```python
from build123d import *

# Parameters (mm, degrees)
SKETCH1_W           = 34
SKETCH1_H           = 30
BOSS_EXTRUDE1_DEPTH = 22.2
CUT_EXTRUDE1_DEPTH  = 51.486037674
SKETCH3_R           = 4
CUT_EXTRUDE2_DEPTH  = 51.486037674


with BuildPart() as part:
    # Sketch1 → Boss-Extrude1 (new body)
    with BuildSketch(Plane(origin=(0, 0, 0), x_dir=(1, 0, 0), z_dir=(0, 1, 0))):
        with Locations((17, 15)):
            Rectangle(SKETCH1_W, SKETCH1_H)
    extrude(amount=BOSS_EXTRUDE1_DEPTH)

    # Sketch2 → Cut-Extrude1 (cut, through all)
    with BuildSketch(Plane.XY):
        Polygon((34, 17.6), (27, 17.6), (23.985037314, 22.2), (34, 22.2), align=None)
        Polygon((0, 22.2), (0, 17.6), (7, 17.6), (10.014962686, 22.2), align=None)
    extrude(amount=-CUT_EXTRUDE1_DEPTH, mode=Mode.SUBTRACT)

    # Sketch3 → Cut-Extrude2 (cut, through all)
    with BuildSketch(Plane.XY):
        with Locations((17, 10.8)):
            Circle(SKETCH3_R)
    extrude(amount=-CUT_EXTRUDE2_DEPTH, mode=Mode.SUBTRACT)


solid = part.part
```
The model under review builds one solid part; all positions refer to its coordinate system, in mm. A direction names the side the tool comes from. Give positions to 0.01 mm unless a question says otherwise; leave off trailing zeros. Loops run counter-clockwise (first coordinate to the right, second up) from the corner with the lowest first, then second, coordinate; pieces in that order, holes last. Notation, with made-up numbers: (49, 25) - (57, 25) arc R8 ccw to (57, 30) - close; hole circle Ø3 at (51, 1). An arc over 180 degrees is marked (long way). Answer as a JSON object with one key per item and string values.
Q1. Insertion check: pin 1 (4 mm diameter, centred on x = 18, y = 11.5, fed in from -Z); pin 2 (8 mm diameter, centred on x = 5, z = -3.5, fed in from +Y); pin 3 (7.5 mm diameter, centred on x = 32, z = -9.5, fed in from +Y); pin 4 (5.5 mm diameter, centred on x = 4.5, z = -7.5, fed in from +Y). Each pin has a flat end and moves straight along its axis. Give the tip position at first contact, or say it passes through.
Worked out:
{"pin 1": "passes through", "pin 2": "stops at y = 20.65", "pin 3": "stops at y = 17.6", "pin 4": "stops at y = 17.98"}
Q2. Mouldability with a two-part tool opening along X and no side actions: class faces 4 (the flat face through (17, 6, -30)), 5 (the flat face through (25.51, 19.87, -14.79)), 6 (the cylindrical face through (14.05, 13.5, -14.79)), 7 (the flat face through (8.49, 19.87, -14.79)) as +X half, -X half, draft (parallel to the pull), parting line (faces both ways), or undercut.
Worked out:
{"face 4": "draft", "face 5": "+X half", "face 6": "undercut", "face 7": "-X half"}
Q3. Add section A-A on x = 17. State the section outline as (y, z) points.
Worked out:
{"outline": "(0, -30) - (6.8, -30) - (6.8, 0) - (0, 0) - close; (14.8, -30) - (22.2, -30) - (22.2, 0) - (14.8, 0) - close"}
Q4. Add section D-D on y = 20.5. State the section outline as (x, z) points.
Worked out:
{"outline": "(8.9, -30) - (25.1, -30) - (25.1, 0) - (8.9, 0) - close"}
Q5. To check wall thickness, follow line 1 along Y through (x, z) = (17, -9); line 2 along X through (y, z) = (11, -8.5) (3 decimals); line 3 along Y through (x, z) = (27.5, -23.5). State the ranges of each line that lie inside material, in increasing order.
Worked out:
{"line 1": "y = 0 to 6.8, 14.8 to 22.2", "line 2": "x = 0 to 13.005, 20.995 to 34", "line 3": "y = 0 to 17.6"}
Q6. Add section C-C on y = 10.8. State the section outline as (x, z) points.
Worked out:
{"outline": "(0, -30) - (13, -30) - (13, 0) - (0, 0) - close; (21, -30) - (34, -30) - (34, 0) - (21, 0) - close"}
Q7. For faces 1 (the flat face through (3, 17.6, -15)), 2 (the flat face through (34, 9, -15)), 3 (the flat face through (31, 17.6, -15)), list the 3-axis set-ups (+Z, -Z, +X, -X, +Y, -Y) from which the entire face can be reached by the end or side of a thin tool; tool diameter is ignored.
Worked out:
{"face 1": "+Z, -Z, -X, +Y", "face 2": "+Z, -Z, +X, +Y, -Y", "face 3": "+Z, -Z, +X, +Y"}
Q8. Add section B-B on z = -11. State the section outline as (x, y) points, plus the area to 3 significant figures.
Worked out:
{"outline": "(0, 0) - (34, 0) - (34, 17.6) - (27, 17.6) - (23.99, 22.2) - (10.01, 22.2) - (7, 17.6) - (0, 17.6) - close; hole circle Ø8 at (17, 10.8)", "area": "626 mm^2"}
